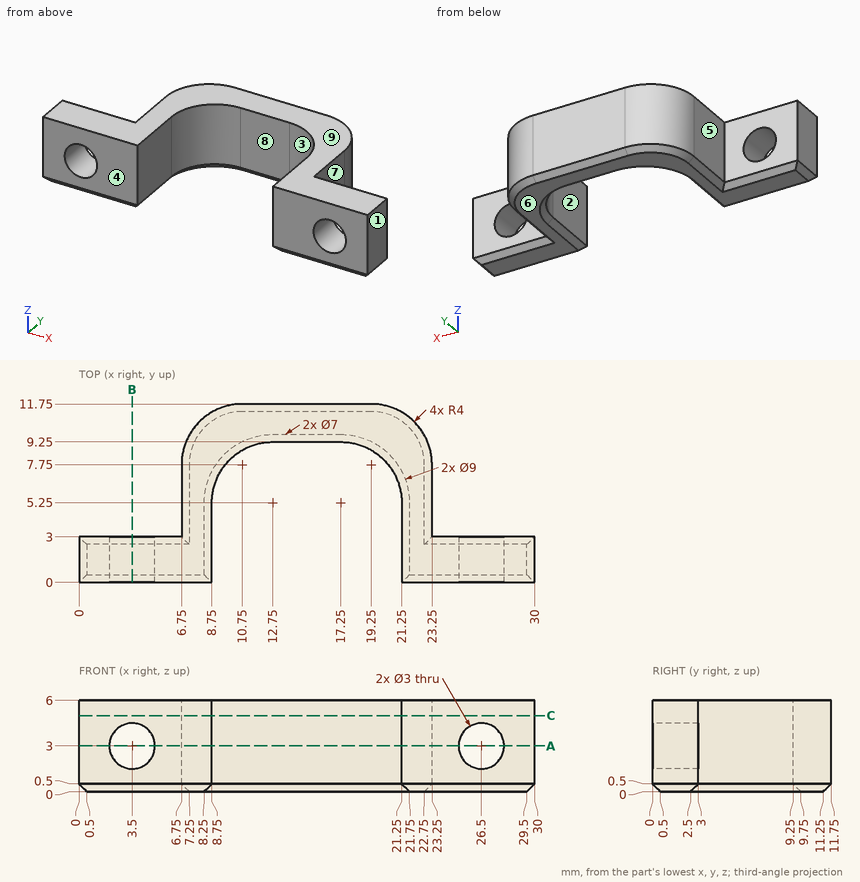
Print and shaded views of the part. All mm, measured from the part's lowest x, y and z. A direction names the side the tool comes from. Give positions to 0.01 mm unless a question says otherwise; leave off trailing zeros. Loops run counter-clockwise (first coordinate to the right, second up) from the corner with the lowest first, then second, coordinate; pieces in that order, holes last.
1) Tool access for the marked faces 5, 6, 7, 8 and 9: list every direction of +Z, -Z, +X, -X, +Y, -Y with a clear straight run to the whole face (end or side of a thin tool).
2) Saw through at B-B (x = 3.5). Write the cut outline in (y, z), plus the area to 3 significant figures.
3) Flat gauge pins, fed straight in: pin 1 Ø1.8 at (x, z) = (3.5, 3) entering from -Y; pin 2 Ø3 at (x, z) = (4, 2.5) entering from +Y; pin 3 Ø2.5 at (y, z) = (5, 4) entering from +X; pin 4 Ø1.4 at (x, z) = (15, 2) entering from -Y. Where does each tip first touch, or does it go through?
4) Saw through at C-C (z = 5). Write the cut outline in (x, y), plus the area to 3 significant figures.
5) Wall check: line 1 (X direction, y = 2.75, z = 2.95); line 2 (Z direction, x = 26.5, y = 1.6); line 3 (Y direction, x = 28, z = 4.7). Give the ranges that are in metal, low to high.
6) Pull direction X, two halves, no side cores. Call the marked faces 1, 2, 3 and 4: +X half, -X half, draft (parallel to the pull), parting line (faces both ways), or undercut.
7) Saw through at A-A (z = 3). Write the cut outline in (x, y), plus the area to 3 significant figures.
Answer block:
1. face 5: +Z, -Z, -X, +Y
1. face 6: -Z, +X, -X, +Y, -Y
1. face 7: +Z, -Z, +X, +Y
1. face 8: +Z, -Z, -Y
1. face 9: +Z, +X, -X, +Y, -Y
2. outline: (0, 0.5) - (0.5, 0) - (2.5, 0) - (3, 0.5) - (3, 1.5) - (0, 1.5) - close; (0, 4.5) - (3, 4.5) - (3, 6) - (0, 6) - close
2. area: 8.75 mm2
3. pin 1: passes through
3. pin 2: stops at y = 3
3. pin 3: stops at x = 23.25
3. pin 4: stops at y = 9.25
4. outline: (0, 0) - (8.75, 0) - (8.75, 5.25) arc R4 cw to (12.75, 9.25) - (17.25, 9.25) arc R4 cw to (21.25, 5.25) - (21.25, 0) - (30, 0) - (30, 3) - (23.25, 3) - (23.25, 7.75) arc R4 ccw to (19.25, 11.75) - (10.75, 11.75) arc R4 ccw to (6.75, 7.75) - (6.75, 3) - (0, 3) - close
4. area: 119 mm2
5. line 1: x = 0 to 2, 5 to 8.75, 21.25 to 25, 28 to 30
5. line 2: z = 0 to 1.5, 4.5 to 6
5. line 3: y = 0 to 3
6. face 1: +X half
6. face 2: undercut
6. face 3: undercut
6. face 4: draft
7. outline: (0, 0) - (2, 0) - (2, 3) - (0, 3) - close; (5, 0) - (8.75, 0) - (8.75, 5.25) arc R4 cw to (12.75, 9.25) - (17.25, 9.25) arc R4 cw to (21.25, 5.25) - (21.25, 0) - (25, 0) - (25, 3) - (23.25, 3) - (23.25, 7.75) arc R4 ccw to (19.25, 11.75) - (10.75, 11.75) arc R4 ccw to (6.75, 7.75) - (6.75, 3) - (5, 3) - close; (28, 0) - (30, 0) - (30, 3) - (28, 3) - close
7. area: 101 mm2
